CAD build for the part. Positions are in the model's coordinates, mm. A direction names the side the tool comes from. Round coordinates to 2 decimals unless told otherwise and drop trailing zeros. Loops run counter-clockwise (first coordinate to the right, second up) from the corner with the lowest first, then second, coordinate; pieces in that order, holes last. Notation, with made-up numbers: M 8,25.25 L 44,25.25 A20 ccw 44,63.25 Z; hole C 15.5,-5 d11. An arc over 180 degrees is marked long. Use a Markdown table: item, result. Add a question column.
(1) Which spindle directions (+Z, -Z, +X, -X, +Y, -Y) get a long thin tool onto all of the face, cutting with end or side? Do faces 4 (the face through (9.918, 0, -1)), 5 (the face through (5, 0, 4.328)), 6 (the face through (1.118, -1, -7)). Say none if no direction does.
(2) Flat gauge pins, fed straight in: P1, Ø0.6, axis at y = 1, z = 5.5, coming from the -X side; P2, Ø2, axis at y = 0, z = -7.42, coming from the -X side; P3, Ø3.5, axis at y = 0, z = -8, coming from the +X side; P4, Ø1, axis at y = 0, z = -7.42, coming from the -X side. Where does each tip first touch, or does it go through?
(3) Band-saw the part on C-C, the plane y = 0.25. Give the number of separate pieces and of enclosed holes in the cut face, and give its area (3 significant figures).
(4) Two-plate mould, pull along Z, no slides. Class faces 1 (the face through (3, 0, 5.778)), 2 (the face through (-7.732, -1, -7)), 3 (the face through (5, 0, -5.522)): released by +Z, released by -Z, zero draft, split by the parting line, or undercut.
(5) Band-saw the part on A-A, the plane x = 7. Write the cut outline in (y, z).
(6) Band-saw the part on B-B, the plane z = -7.5. Write the cut outline in (x, y).
(7) Wall check: L1, parallel to Z at x = 3.75, y = 1.5; L2, parallel to Y at x = -5.75, z = -0.25; L3, parallel to X at y = -1, z = 5.25. Give the ranges that are in metal, low to high.
(8) Band-saw the part on D-D, the plane z = 1.5. Write the cut outline in (x, y).
from build123d import *

# Parameters (mm, degrees)
BOSS_EXTRUDE1_DEPTH      = 3
BOSS_EXTRUDE1_DEPTH_BACK = 3
BOSS_EXTRUDE2_DEPTH      = 2
BOSS_EXTRUDE2_DEPTH_BACK = 2
BOSS_EXTRUDE3_DEPTH      = 3.2
BOSS_EXTRUDE3_DEPTH_BACK = 3.2
SKETCH3_R                = 1.25
CUT_EXTRUDE1_DEPTH       = 1.2
CUT_EXTRUDE1_DEPTH_BACK  = 7.2
BOSS_EXTRUDE4_DEPTH      = 3
BOSS_EXTRUDE4_DEPTH_BACK = 3
SKETCH6_W                = 0.6
SKETCH6_H                = 4
BOSS_EXTRUDE5_DEPTH      = 1.6
BOSS_EXTRUDE5_DEPTH_BACK = 1.6
FILLET1_R                = 0.5
SKETCH7_R                = 0.8
CUT_EXTRUDE2_DEPTH       = 2.5
CUT_EXTRUDE2_DEPTH_BACK  = 21.05


with BuildPart() as part:
    # Sketch1 → Boss-Extrude1 (new body, two sides)
    with BuildSketch(Plane(origin=(0, 0, 0), x_dir=(1, 0, 0), z_dir=(0, 1, 0))) as boss_extrude1_sk:
        with BuildLine():
            Line((-8.832423279, -5.07801101), (0.167576721, -5.07801101))
            Line((0.167576721, -5.07801101), (0.89698899, -4.32801101))
            Line((0.89698899, -4.32801101), (8.917576721, -4.32801101))
            ThreePointArc((8.917576721, -4.32801101), (9.624683502, -4.035117791), (9.917576721, -3.32801101))
            Line((9.917576721, -3.32801101), (9.917576721, 4.62198899))
            ThreePointArc((9.917576721, 4.62198899), (9.771130112, 4.975542381), (9.417576721, 5.12198899))
            Line((9.417576721, 5.12198899), (-9.332423279, 5.12198899))
            ThreePointArc((-9.332423279, 5.12198899), (-9.685976669, 4.975542381), (-9.832423279, 4.62198899))
            Line((-9.832423279, 4.62198899), (-9.832423279, -4.07801101))
            ThreePointArc((-9.832423279, -4.07801101), (-9.53953006, -4.785117791), (-8.832423279, -5.07801101))
        make_face()
    extrude(amount=BOSS_EXTRUDE1_DEPTH)
    extrude(boss_extrude1_sk.sketch, amount=-BOSS_EXTRUDE1_DEPTH_BACK)

    # Sketch2 → Boss-Extrude2 (add, two sides)
    with BuildSketch(Plane(origin=(0, 0, 0), x_dir=(1, 0, 0), z_dir=(0, 1, 0))) as boss_extrude2_sk:
        with BuildLine():
            Line((-6.582423279, -5.07801101), (-6.282423279, -5.07801101))
            Line((-6.282423279, -5.07801101), (-6.282423279, -5.52801101))
            ThreePointArc((-6.282423279, -5.52801101), (-6.209199974, -5.704787705), (-6.032423279, -5.77801101))
            Line((-6.032423279, -5.77801101), (11.717576721, -5.77801101))
            Line((11.717576721, -5.77801101), (11.717576721, -6.07801101))
            Line((11.717576721, -6.07801101), (-6.282423279, -6.07801101))
            Line((-6.282423279, -6.07801101), (-6.332423279, -6.07801101))
            ThreePointArc((-6.332423279, -6.07801101), (-6.509199974, -6.004787705), (-6.582423279, -5.82801101))
            Line((-6.582423279, -5.82801101), (-6.582423279, -5.07801101))
        make_face()
    extrude(amount=BOSS_EXTRUDE2_DEPTH)
    extrude(boss_extrude2_sk.sketch, amount=-BOSS_EXTRUDE2_DEPTH_BACK)

    # Sketch4 → Boss-Extrude3 (add, two sides)
    with BuildSketch(Plane(origin=(0, 0, 0), x_dir=(1, 0, 0), z_dir=(0, 1, 0))) as boss_extrude3_sk:
        with BuildLine():
            Line((-6.832423279, 2.944690743), (-6.832423279, 5.12198899))
            Line((-6.832423279, 5.12198899), (-2.832423279, 5.12198899))
            Line((-2.832423279, 5.12198899), (-2.832423279, 2.944690743))
            ThreePointArc((-2.832423279, 2.944690743), (-4.832423279, 0.944690743), (-6.832423279, 2.944690743))
        make_face()
        with BuildLine():
            Line((6.667576721, 5.12198899), (6.667576721, 2.944690743))
            ThreePointArc((6.667576721, 2.944690743), (4.667576721, 0.944690743), (2.667576721, 2.944690743))
            Line((2.667576721, 2.944690743), (2.667576721, 5.12198899))
            Line((2.667576721, 5.12198899), (6.667576721, 5.12198899))
        make_face()
    extrude(amount=BOSS_EXTRUDE3_DEPTH)
    extrude(boss_extrude3_sk.sketch, amount=-BOSS_EXTRUDE3_DEPTH_BACK)

    # Sketch3 → Cut-Extrude1 (cut, two sides)
    with BuildSketch(Plane(origin=(0, 3, 0), x_dir=(1, 0, 0), z_dir=(0, 1, 0))) as cut_extrude1_sk:
        with Locations((-4.832423279, 2.944690743)):
            Circle(SKETCH3_R)
        with Locations((4.667576721, 2.944690743)):
            Circle(SKETCH3_R)
    extrude(amount=CUT_EXTRUDE1_DEPTH, mode=Mode.SUBTRACT)
    extrude(cut_extrude1_sk.sketch, amount=-CUT_EXTRUDE1_DEPTH_BACK, mode=Mode.SUBTRACT)

    # Sketch5 → Boss-Extrude4 (add, two sides)
    with BuildSketch(Plane(origin=(0, 0, 0), x_dir=(1, 0, 0), z_dir=(0, 1, 0))) as boss_extrude4_sk:
        Polygon((-6.832423279, 5.12198899), (-2.832423279, 5.12198899), (-3.082423279, 5.52198899), (-6.582423279, 5.52198899), align=None)
        Polygon((6.417576721, 5.52198899), (6.667576721, 5.12198899), (2.667576721, 5.12198899), (2.917576721, 5.52198899), align=None)
    extrude(amount=BOSS_EXTRUDE4_DEPTH)
    extrude(boss_extrude4_sk.sketch, amount=-BOSS_EXTRUDE4_DEPTH_BACK)

    # Sketch6 → Boss-Extrude5 (add, two sides)
    with BuildSketch(Plane(origin=(0, 0, 0), x_dir=(1, 0, 0), z_dir=(0, 1, 0))) as boss_extrude5_sk:
        with Locations((-8.032423279, 7.12198899)):
            Rectangle(SKETCH6_W, SKETCH6_H)
        with Locations((0.817576721, 7.12198899)):
            Rectangle(SKETCH6_W, SKETCH6_H)
        with Locations((8.067576721, 7.12198899)):
            Rectangle(SKETCH6_W, SKETCH6_H)
    extrude(amount=BOSS_EXTRUDE5_DEPTH)
    extrude(boss_extrude5_sk.sketch, amount=-BOSS_EXTRUDE5_DEPTH_BACK)

    # Fillet1
    fillet1_edges = [part.edges().sort_by_distance(p)[0] for p in [
        (-8.032423279, -1.6, -9.12198899),
        (-8.032423279, 1.6, -9.12198899),
        (0.817576721, -1.6, -9.12198899),
        (0.817576721, 1.6, -9.12198899),
        (8.067576721, -1.6, -9.12198899),
        (8.067576721, 1.6, -9.12198899),
    ]]
    fillet(fillet1_edges, radius=FILLET1_R)

    # Sketch7 → Cut-Extrude2 (cut, two sides)
    with BuildSketch(Plane.ZY.offset(8.332423279)) as cut_extrude2_sk:
        with Locations((-7.42198899, 0)):
            Circle(SKETCH7_R)
    extrude(amount=CUT_EXTRUDE2_DEPTH, mode=Mode.SUBTRACT)
    extrude(cut_extrude2_sk.sketch, amount=-CUT_EXTRUDE2_DEPTH_BACK, mode=Mode.SUBTRACT)


solid = part.part
Return value:
| question | item | result |
|---|---|---|
| 1 | face 4 | -Z, +X, +Y, -Y |
| 1 | face 5 | +X, +Y, -Y |
| 1 | face 6 | -Z, +Y, -Y |
| 2 | P1 | x = -6.58 |
| 2 | P2 | x = -8.33 |
| 2 | P3 | x = 8.37 |
| 2 | P4 | through |
| 3 | separate pieces | 4 |
| 3 | enclosed holes | 2 |
| 3 | area | 197 mm^2 |
| 4 | face 1 | undercut |
| 4 | face 2 | zero draft |
| 4 | face 3 | released by -Z |
| 5 | outline | M -3,-5.12 L 3,-5.12 L 3,4.33 L -3,4.33 Z; M -2,5.78 L 2,5.78 L 2,6.08 L -2,6.08 Z |
| 6 | outline | M -8.33,-1.6 L -7.73,-1.6 L -7.73,-0.8 L -8.33,-0.8 Z; M -8.33,0.8 L -7.73,0.8 L -7.73,1.6 L -8.33,1.6 Z; M 0.52,-1.6 L 1.12,-1.6 L 1.12,-0.8 L 0.52,-0.8 Z; M 0.52,0.8 L 1.12,0.8 L 1.12,1.6 L 0.52,1.6 Z; M 7.77,-1.6 L 8.37,-1.6 L 8.37,-0.8 L 7.77,-0.8 Z; M 7.77,0.8 L 8.37,0.8 L 8.37,1.6 L 7.77,1.6 Z |
| 7 | L1 | -5.52 to -3.79, -2.1 to 4.33, 5.78 to 6.08 |
| 7 | L2 | -3 to 3 |
| 7 | L3 | -6.58 to -6.28 |
| 8 | outline | M -9.83,-3 L 9.92,-3 L 9.92,3 L -9.83,3 Z |
